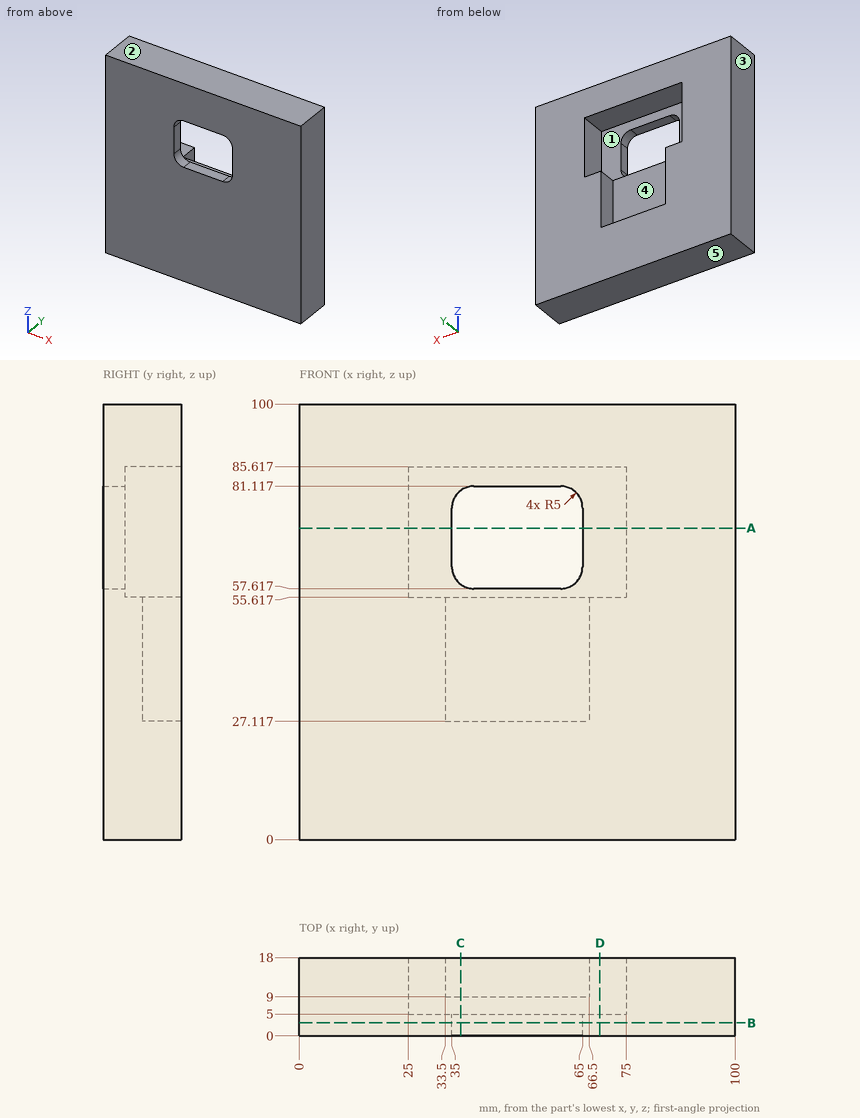
Design review of the part shown in the three views and the two pictorial views. Dimensions are in mm from the part's minimum x, y and z. A direction names the side the tool comes from. Round coordinates to 2 decimals unless told otherwise and drop trailing zeros. Write each loop counter-clockwise with the first axis right and the second up, starting at its lowest first coordinate (ties: lowest second). Pieces come first, ordered by that corner, then holes.
1) Machinability: for the marked faces 1 and 2, which of the approach directions +Z, -Z, +X, -X, +Y, -Y give a long, thin tool a straight path to every point of the face, cutting with its end or side? Answer none if there is none.
Answer below:
face 1: +Y
face 2: +Z, +X, -X, +Y, -Y
2) Take a section at D-D on x = 69. Give the boundary of the cut face in (y, z), then the cut area to 3 significant figures.
Answer below:
outline: (0, 0) - (18, 0) - (18, 55.62) - (5, 55.62) - (5, 85.62) - (18, 85.62) - (18, 100) - (0, 100) - close
area: 1,410 mm2
3) Mouldability with a two-part tool opening along X and no side actions: class the marked faces 3, 4 and 5 as +X half, -X half, draft (parallel to the pull), parting line (faces both ways), or undercut.
Answer below:
face 3: -X half
face 4: undercut
face 5: draft
4) Take a section at B-B on y = 3. Give the boundary of the cut face in (x, z), then the cut area to 3 significant figures.
Answer below:
outline: (0, 0) - (100, 0) - (100, 100) - (0, 100) - close; hole (35, 62.62) arc R5 ccw to (40, 57.62) - (60, 57.62) arc R5 ccw to (65, 62.62) - (65, 76.12) arc R5 ccw to (60, 81.12) - (40, 81.12) arc R5 ccw to (35, 76.12) - close
area: 9,320 mm2
5) Take a section at A-A on z = 71.5. Give the boundary of the cut face in (x, y).
Answer below:
outline: (0, 0) - (35, 0) - (35, 5) - (25, 5) - (25, 18) - (0, 18) - close; (65, 0) - (100, 0) - (100, 18) - (75, 18) - (75, 5) - (65, 5) - close
6) For line 1 along X through (y, z) = (2.5, 63.5); line 2 along Z through (x, y) = (27, 6.75); line 3 along X through (y, z) = (13, 62), list the stretches that pass through material, from the lowest coordinate up.
Answer below:
line 1: x = 0 to 35, 65 to 100
line 2: z = 0 to 55.62, 85.62 to 100
line 3: x = 0 to 25, 75 to 100
7) Insertion check: pin 1 Ø23 at (x, z) = (51.5, 41) entering from +Y; pin 2 Ø15 at (x, z) = (53, 77.5) entering from +Y. Each pin has a flat end and moves straight along its axis. Give the tip position at first contact, or say it passes through.
Answer below:
pin 1: stops at y = 9
pin 2: stops at y = 5
8) Take a section at C-C on x = 37. Give the boundary of the cut face in (y, z), then the cut area to 3 significant figures.
Answer below:
outline: (0, 0) - (18, 0) - (18, 27.12) - (9, 27.12) - (9, 55.62) - (5, 55.62) - (5, 58.62) - (0, 58.62) - close; (0, 80.12) - (5, 80.12) - (5, 85.62) - (18, 85.62) - (18, 100) - (0, 100) - close
area: 1,050 mm2
